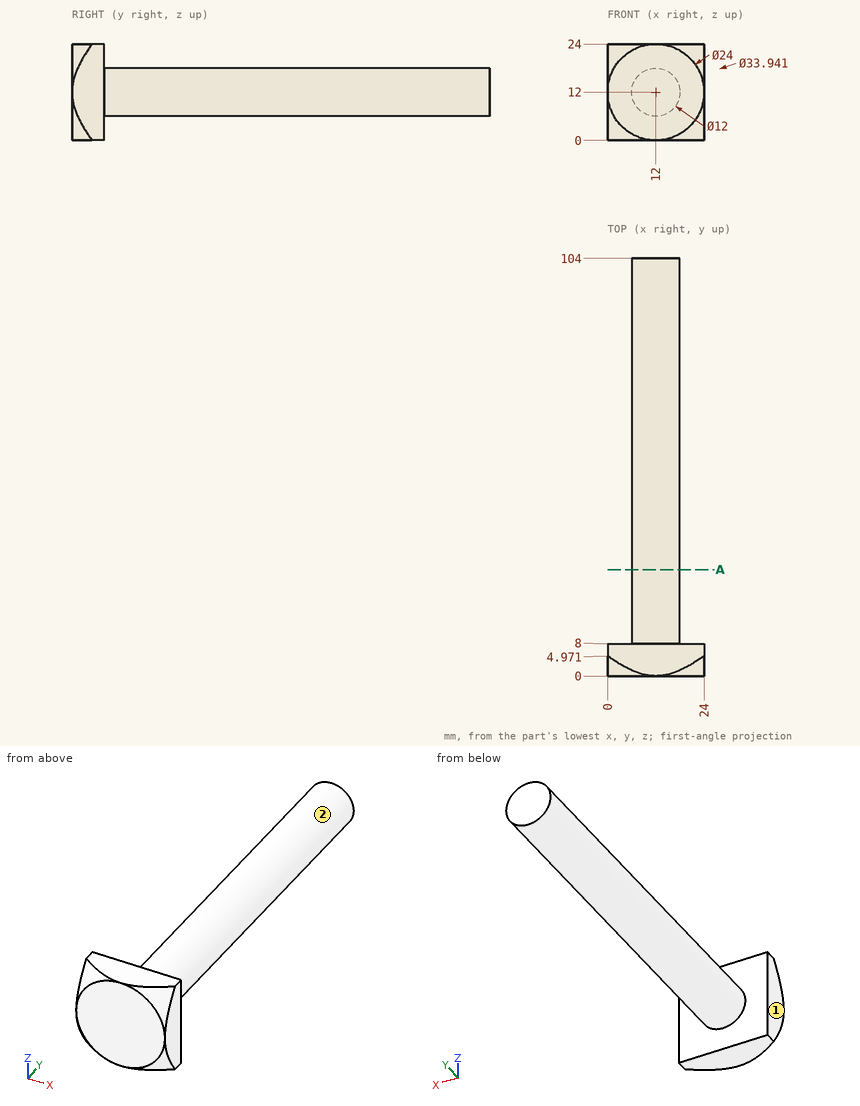
Part print with two shaded views. Sizes in mm from the minimum x, y, z corner. A direction names the side the tool comes from. Coordinates: 2 decimals unless noted, no trailing zeros. Order: outer loops, then holes, each group sorted by start corner. A loop starts at its lowest first (then second) coordinate and runs counter-clockwise, first axis right, second up. Notation, with made-up numbers: (85.25, 28) - (105.25, 28) arc R15 cw to (105.25, 56) - close; hole circle Ø5 at (46.5, 28). An arc over 180 degrees is marked (long way). Write item = value, one per line. Start each with the question number.
1) Saw through at A-A on y = 26.5. Write the cut outline in (x, z).
2) Flat gauge pins, fed straight in: pin 1 Ø10 at (x, y) = (18, 73) entering from +Z; pin 2 Ø3 at (y, z) = (68, 17) entering from +X; pin 3 Ø2 at (x, z) = (20, 15) entering from +Y. Where does each tip first touch, or does it go through?
3) Wall check: line 1 along Y through (x, z) = (17.5, 7.25); line 2 along Z through (x, y) = (12.25, 86) (1 decimal); line 3 along Z through (x, y) = (16, 43). Give the ranges that are in metal, low to high. Write a range as from..to.
4) 3-axis set-ups, long thin cutter, end or side, ignore diameter. For the marked faces 1 and 2: which of +Z, -Z, +X, -X, +Y, -Y reach the whole face in a straight line?
From the geometry:
q1.outline = circle Ø12 at (12, 12)
q2.pin_1 = 17.92
q2.pin_2 = 16.87
q2.pin_3 = 8
q3.line_1 = 0..8
q3.line_2 = 6..18
q3.line_3 = 7.53..16.47
q4.face_1 = +Z, -Z, -X, +Y, -Y
q4.face_2 = +Y
